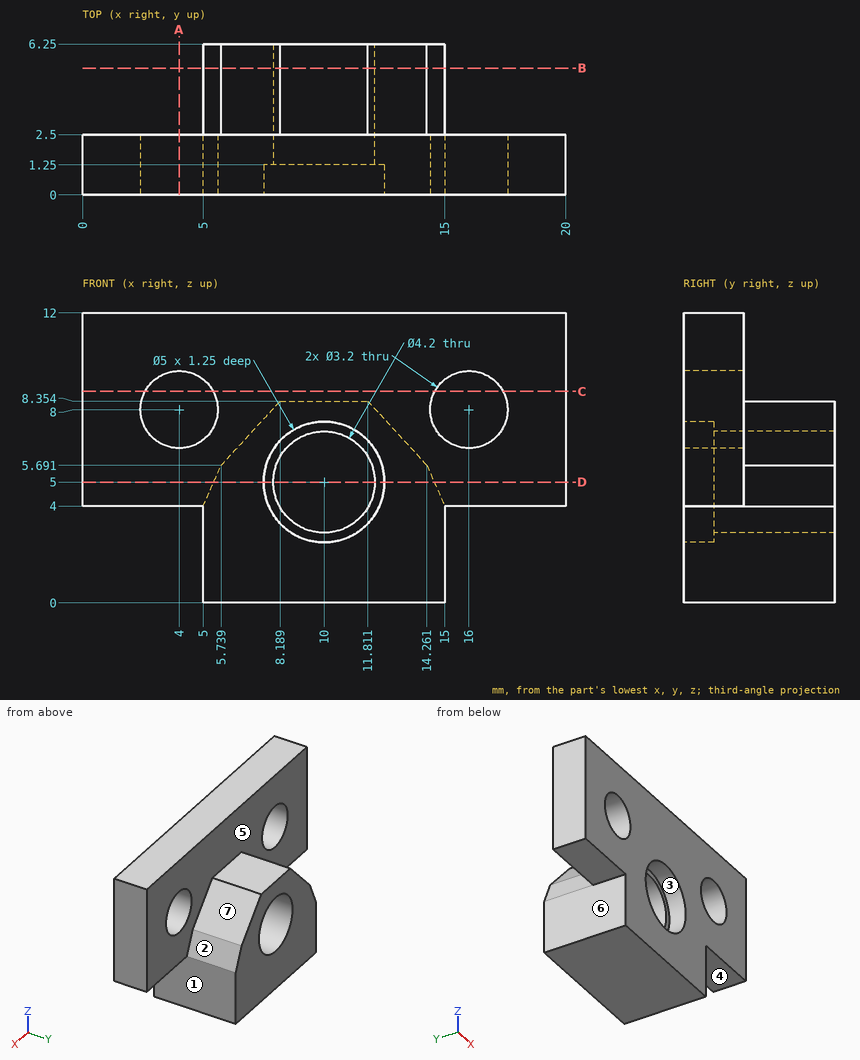
Geometry check sheet. Reference: drawing and pictorial views, mm from the part's lowest x, y, z. A direction names the side the tool comes from. Give positions to 0.01 mm unless a question says otherwise; leave off trailing zeros. Order: outer loops, then holes, each group sorted by start corner. A loop starts at its lowest first (then second) coordinate and runs counter-clockwise, first axis right, second up. Notation, with made-up numbers: M 10.5,49.5 L 63.5,49.5 A22 ccw 63.5,73.5 Z; hole C -7.75,-28.75 d3. An arc over 180 degrees is marked long. Answer in a Markdown table with one row per item. Add a question column.
Q1. Gauge pin test, flat ends, axial feed: pin 1 Ø4 at (x, z) = (10, 5) entering from +Y; pin 2 Ø4 at (x, z) = (16.5, 7) entering from -Y; pin 3 Ø1.1 at (x, y) = (10, 5) entering from +Z; pin 4 Ø1.2 at (y, z) = (3, 1.5) entering from +X. Record the tip position at first contact, or that the pin passes through.
Q2. Access from +Z, -Z, +X, -X, +Y, -Y to the whole of each face (thin tool, end or side, straight path). Record for the marked faces 5, 6 and 7.
Q3. Thickness scan on L1, parallel to Z at x = 4, y = 1.5; L2, parallel to X at y = 0.8, z = 5; L3, parallel to X at y = 1.95, z = 8. Record the ranges inside material, lowest first.
Q4. Release check for a two-part mould opening along Z. For the marked faces 1, 2, 3 and 4 record: released by +Z, released by -Z, zero draft, split by the parting line, or undercut.
Q5. Sectioned sample at A-A, the plane x = 4. Record the boundary of the cut face in (y, z), and give its area (3 significant figures).
Q6. Sectioned sample at D-D, the plane z = 5. Record the boundary of the cut face in (x, y).
Q7. Sectioned sample at B-B, the plane y = 5.25. Record the boundary of the cut face in (x, z), and give its area (3 significant figures).
Q8. Sectioned sample at C-C, the plane z = 8.75. Record the boundary of the cut face in (x, y).
Verdict:
| question | item | result |
|---|---|---|
| 1 | pin 1 | through |
| 1 | pin 2 | y = 0 |
| 1 | pin 3 | z = 8.35 |
| 1 | pin 4 | x = 15 |
| 2 | face 5 | +Z, +Y |
| 2 | face 6 | -Z, -X, +Y, -Y |
| 2 | face 7 | +Z, +X, +Y |
| 3 | L1 | 4 to 6.4, 9.6 to 12 |
| 3 | L2 | 0 to 7.5, 12.5 to 20 |
| 3 | L3 | 0 to 2.4, 5.6 to 14.4, 17.6 to 20 |
| 4 | face 1 | zero draft |
| 4 | face 2 | released by +Z |
| 4 | face 3 | undercut |
| 4 | face 4 | released by -Z |
| 5 | outline | M 0,4 L 2.5,4 L 2.5,6.4 L 0,6.4 Z; M 0,9.6 L 2.5,9.6 L 2.5,12 L 0,12 Z |
| 5 | area | 12.0 mm² |
| 6 | outline | M 0,0 L 7.5,0 L 7.5,1.25 L 7.9,1.25 L 7.9,6.25 L 5.44,6.25 L 5.44,2.5 L 0,2.5 Z; M 12.1,1.25 L 12.5,1.25 L 12.5,0 L 20,0 L 20,2.5 L 14.56,2.5 L 14.56,6.25 L 12.1,6.25 Z |
| 7 | outline | M 5,0 L 15,0 L 15,4 L 14.26,5.69 L 11.81,8.35 L 8.19,8.35 L 5.74,5.69 L 5,4 Z; hole C 10,5 d4.2 |
| 7 | area | 58.0 mm² |
| 8 | outline | M 0,0 L 2.59,0 L 2.59,2.5 L 0,2.5 Z; M 5.41,0 L 14.59,0 L 14.59,2.5 L 5.41,2.5 Z; M 17.41,0 L 20,0 L 20,2.5 L 17.41,2.5 Z |
